from build123d import *
from build123d import SkipClean  # not in build123d's __all__

# Parameters (mm, degrees)
F0_R     = 5
F1_DEPTH = 25


with BuildPart() as f1:
    # F0 (on Front) → F1 (new body)
    with BuildSketch(Plane.XZ):
        with BuildLine():
            ThreePointArc((-15, 40), (-10.6066017178, 50.6066017178), (0, 55))
            Line((0, 55), (0, 60))
            ThreePointArc((0, 60), (-5, 65), (0, 70))
            Line((0, 70), (0, 75))
            ThreePointArc((0, 75), (-24.7487373415, 64.7487373415), (-35, 40))
            Line((-35, 40), (-35, 0))
            Line((-35, 0), (-30, 0))
            ThreePointArc((-30, 0), (-25, 5), (-20, 0))
            Line((-20, 0), (-15, 0))
            Line((-15, 0), (-15, 40))
        make_face()
        with Locations((-25, 20)):
            Circle(F0_R, mode=Mode.SUBTRACT)
        with Locations((-25, 40)):
            Circle(F0_R, mode=Mode.SUBTRACT)
        with Locations((-17.6776695297, 57.6776695297)):
            Circle(F0_R, mode=Mode.SUBTRACT)
    extrude(amount=F1_DEPTH)

    # F2: F1 across plane


with BuildPart() as f1_1:
    add(f1.part, clean=False)
    with SkipClean():  # cleaning this boolean's faces spoils the solid; the shape is the same uncleaned
        add(f1.part.mirror(Plane.YZ), clean=False)

    # F3: F1 across plane


with BuildPart() as f1_2:
    add(f1_1.part, clean=False)
    add(f1_1.part.mirror(Plane.XY), clean=False)


solid = f1_2.part
The listing builds one solid part. Answer for the finished solid, in the listing's coordinates (mm). A direction names the side the tool comes from. Round coordinates to 2 decimals unless told otherwise and drop trailing zeros. Order: outer loops, then holes, each group sorted by start corner. A loop starts at its lowest first (then second) coordinate and runs counter-clockwise, first axis right, second up. Notation, with made-up numbers: (11.5, 25.5) - (54.5, 25.5) arc R21 cw to (54.5, 42.5) - close; hole circle Ø2 at (55.25, 59). An arc over 180 degrees is marked (long way). Write item = value, one per line. Start each with the question number.
1) Section D-D, the plane x = 16.5 is taken. Write down the section's boundary in (y, z), plus the area to 3 significant figures.
2) Section A-A, the plane z = -20 is taken. Write down the section's boundary in (x, y).
3) Section C-C, the plane z = 65 is taken. Write down the section's boundary in (x, y), plus the area to 3 significant figures.
4) For a pull along X with two mould halves and no side action, classify faces 3 (the flat face through (16, 0, -1)), 4 (the cylindrical face through (-25.651, -12.325, 44.957)) as released by +X, released by -X, zero draft, split by the parting line, or undercut.
5) Straight lines are drawn through the part: L1, parallel to Z at x = 0, y = -8.25; L2, parallel to X at y = -10.25, z = -20; L3, parallel to Z at x = -29, y = -3. For each, find the intervals that lie inside material, in ascending order.
6) For faces 1 (the flat face through (15, -12, 1)), 2 (the flat face through (16, -25, -1)), determine the directions among +Z, -Z, +X, -X, +Y, -Y from which every point of the face is accessible in a straight line to the end or side of a thin tool.
7) Given pin 1 (1.5 mm diameter, centred on x = -26.5, y = -5, fed in from -Z); pin 2 (3 mm diameter, centred on x = -13.5, y = -11.5, fed in from +Z); pin 3 (12 mm diameter, centred on x = -23.5, y = -4, fed in from +Z), each flat-ended and moving along its own axis, determine where each tip first touches the part or whether it passes through.
8) Section B-B, the plane x = 26.5 is taken. Write down the section's boundary in (y, z), plus the area to 3 significant figures.
Results list:
q1.outline = (-25, -70.87) - (0, -70.87) - (0, -62.54) - (-25, -62.54) - close; (-25, -52.82) - (0, -52.82) - (0, 52.82) - (-25, 52.82) - close; (-25, 62.54) - (0, 62.54) - (0, 70.87) - (-25, 70.87) - close
q1.area = 3,060 mm^2
q2.outline = (-35, -25) - (-30, -25) - (-30, 0) - (-35, 0) - close; (-20, -25) - (-15, -25) - (-15, 0) - (-20, 0) - close; (15, -25) - (20, -25) - (20, 0) - (15, 0) - close; (30, -25) - (35, -25) - (35, 0) - (30, 0) - close
q3.outline = (-24.49, -25) - (-5, -25) - (-5, 0) - (-24.49, 0) - close; (5, -25) - (24.49, -25) - (24.49, 0) - (5, 0) - close
q3.area = 975 mm^2
q4.face_3 = zero draft
q4.face_4 = undercut
q5.L1 = -75 to -70, -60 to -55, 55 to 60, 70 to 75
q5.L2 = -35 to -30, -20 to -15, 15 to 20, 30 to 35
q5.L3 = -59.6 to -43, -37 to -23, -17 to -3, 3 to 17, 23 to 37, 43 to 59.6
q6.face_1 = +Y, -Y
q6.face_2 = +Z, -Z, +X, -X, -Y
q7.pin_1 = -63.71
q7.pin_2 = 72.88
q7.pin_3 = 70.31
q8.outline = (-25, -62.86) - (0, -62.86) - (0, -44.77) - (-25, -44.77) - close; (-25, -35.23) - (0, -35.23) - (0, -24.77) - (-25, -24.77) - close; (-25, -15.23) - (0, -15.23) - (0, -4.77) - (-25, -4.77) - close; (-25, 4.77) - (0, 4.77) - (0, 15.23) - (-25, 15.23) - close; (-25, 24.77) - (0, 24.77) - (0, 35.23) - (-25, 35.23) - close; (-25, 44.77) - (0, 44.77) - (0, 62.86) - (-25, 62.86) - close
q8.area = 1,950 mm^2
